```python
from build123d import *

# Parameters (mm, degrees)
F1_DEPTH = 31.75
F2_R     = 1.27
F3_R     = 6.35
F4_DEPTH = 50.8


with BuildPart() as f1:
    # F0 (on Front) → F1 (new body)
    with BuildSketch(Plane.XZ):
        with BuildLine():
            ThreePointArc((-65.460752, 2.190165), (-65.764729, 0.798677), (-64.585426, 0))
            Line((-64.585426, 0), (51.586725, 0))
            Line((51.586725, 0), (51.586725, 27.440994))
            ThreePointArc((51.586725, 27.440994), (51.109575, 28.433107), (50.036663, 28.679729))
            Line((50.036663, 28.679729), (-64.717408, 2.73533))
            ThreePointArc((-64.717408, 2.73533), (-64.735903, 2.729636), (-64.753319, 2.721199))
            ThreePointArc((-64.753319, 2.721199), (-65.122522, 2.476312), (-65.460752, 2.190165))
        make_face()
    extrude(amount=F1_DEPTH)

    # F2
    f2_edges = [f1.edges().sort_by_distance(p)[0] for p in [
        (51.586725, -15.875, 0),
    ]]
    fillet(f2_edges, radius=F2_R)

    # F3 (on face) → F4 (cut)
    with BuildSketch(Plane.YZ.offset(51.586725)):
        with Locations((-15.875, 14.355497)):
            Circle(F3_R)
    extrude(amount=-F4_DEPTH, mode=Mode.SUBTRACT)


solid = f1.part
```
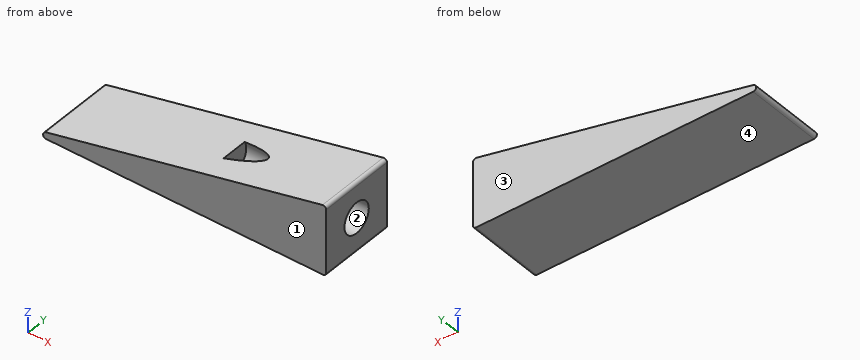
Here's how the part is built. I have some questions about the finished solid (model axes, mm). Face numbers are marked on the shaded views. Round coordinates to 2 decimals unless told otherwise and drop trailing zeros. Write each loop counter-clockwise with the first axis right and the second up, starting at its lowest first coordinate (ties: lowest second). Pieces come first, ordered by that corner, then holes.
Q1. Please list where these lines run through material, in increasing order: probe 1 along Z at (x, y) = (20, -20.5); probe 2 along Z at (x, y) = (37, -12); probe 3 along Y at (x, z) = (8.5, 11.5).
Q2. Will these pins go through, and if not, where does the flat tip stop? P1, Ø8, axis at x = 21, z = 25, coming from the +Y side; P2, Ø5, axis at x = 39, y = -20.5, coming from the +Z side; P3, Ø11.5, axis at y = -15.88, z = 14.36, coming from the +X side; P4, Ø1, axis at x = -34.5, y = -14.5, coming from the +Z side.
Q3. If we mould it in two halves opening along Y, with no side actions, what happens to the marked faces 1, 2, 3 and 4? For each: +Y half, -Y half, draft (parallel to the pull), parting line (faces both ways), or undercut.
Q4. If we section it at B-B on z = 19.5: Write out the boundary of the cut face in (x, y), plus the area to 3 significant figures.
Answer below:
1. probe 1: z = 0 to 10, 18.71 to 21.89
1. probe 2: z = 0 to 9.32, 19.39 to 25.73
1. probe 3: y = -31.75 to -21.55, -10.2 to 0
2. P1: stops at y = 0
2. P2: stops at z = 26.75
2. P3: stops at x = 0.79
2. P4: stops at z = 9.68
3. face 1: -Y half
3. face 2: undercut
3. face 3: +Y half
3. face 4: draft
4. outline: (9.43, -31.75) - (51.59, -31.75) - (51.59, -19.6) - (9.43, -19.6) - close; (9.43, -12.15) - (51.59, -12.15) - (51.59, 0) - (9.43, 0) - close
4. area: 1,020 mm2
